from build123d import *

# Parameters (mm, degrees)
SKETCH1_R                      = 25
BOSS_EXTRUDE1_DEPTH            = 10.8
BOSS_EXTRUDE2_START            = 2
SKETCH2_R                      = 31.25
BOSS_EXTRUDE2_DEPTH            = 2
BOSS_EXTRUDE3_START            = 2.5
SKETCH3_R                      = 31.25
SKETCH3_R_2                    = 30.1
SKETCH3_R_3                    = 19.9
BOSS_EXTRUDE3_DEPTH            = 2.5
CUT_EXTRUDE1_START             = -0.4
SKETCH4_R                      = 31.25
SKETCH4_R_2                    = 27.4
CUT_EXTRUDE1_DEPTH             = 0.4
CUT_EXTRUDE2_START             = -2.5
SKETCH5_R                      = 25
SKETCH5_R_2                    = 19.9
CUT_EXTRUDE2_DEPTH             = 2.5
FILLET1_R                      = 0.2
CUT_EXTRUDE3_REACH             = 67.733
SKETCH7_R                      = 2.15
CUT_EXTRUDE3_DIRECTION_2_DEPTH = 66.732526195
CUT_EXTRUDE4_DEPTH             = 66.732526212
CUT_EXTRUDE4_DEPTH_BACK        = 16
SKETCH8_R                      = 4.15


with BuildPart() as part:
    # Sketch1 → Boss-Extrude1 (new body)
    with BuildSketch(Plane(origin=(0, 0, 0), x_dir=(1, 0, 0), z_dir=(0, 1, 0))):
        with Locations(Location((0, 0, 0), (0, 0, 90))):
            Circle(SKETCH1_R)
        with BuildLine():
            Line((-2.5, 2), (0.5, 2))
            ThreePointArc((0.5, 2), (-1, -2.5), (-2.5, 2))
        make_face(mode=Mode.SUBTRACT)
    extrude(amount=BOSS_EXTRUDE1_DEPTH)

    # Sketch2 → Boss-Extrude2 (add)
    with BuildSketch(Plane.XZ.offset(BOSS_EXTRUDE2_START)):
        with Locations(Location((-1, 0, 0), (0, 0, 270))):
            Circle(SKETCH2_R)
        with BuildLine():
            Line((0.5, -2), (-2.5, -2))
            ThreePointArc((-2.5, -2), (-1, 2.5), (0.5, -2))
        make_face(mode=Mode.SUBTRACT)
    extrude(amount=-BOSS_EXTRUDE2_DEPTH)

    # Sketch3 → Boss-Extrude3 (add)
    # profile 1 of 2: a face of its own
    with BuildSketch(Plane.XZ.offset(2).offset(BOSS_EXTRUDE3_START)):
        with Locations(Location((-1, 0, 0), (0, 0, 270))):
            Circle(SKETCH3_R)
        with Locations(Location((-1, 0, 0), (0, 0, 270))):
            Circle(SKETCH3_R_2, mode=Mode.SUBTRACT)
    # profile 2 of 2: a face of its own
    with BuildSketch(Plane.XZ.offset(2).offset(BOSS_EXTRUDE3_START)):
        with Locations(Location((-1, 0, 0), (0, 0, 270))):
            Circle(SKETCH3_R_3)
        with BuildLine():
            Line((0.5, -2), (-2.5, -2))
            ThreePointArc((-2.5, -2), (-1, 2.5), (0.5, -2))
        make_face(mode=Mode.SUBTRACT)
    extrude(amount=-BOSS_EXTRUDE3_DEPTH)

    # Sketch4 → Cut-Extrude1 (cut)
    with BuildSketch(Plane(origin=(0, 0, 0), x_dir=(1, 0, 0), z_dir=(0, 1, 0)).offset(CUT_EXTRUDE1_START)):
        with Locations(Location((-1, 0, 0), (0, 0, 270))):
            Circle(SKETCH4_R)
        with Locations(Location((0, 0, 0), (0, 0, 270))):
            Circle(SKETCH4_R_2, mode=Mode.SUBTRACT)
    extrude(amount=CUT_EXTRUDE1_DEPTH, mode=Mode.SUBTRACT)

    # Sketch5 → Cut-Extrude2 (cut)
    with BuildSketch(Plane(origin=(0, 10.8, 0), x_dir=(1, 0, 0), z_dir=(0, 1, 0)).offset(CUT_EXTRUDE2_START)):
        with Locations(Location((0, 0, 0), (0, 0, 90))):
            Circle(SKETCH5_R)
        with Locations(Location((-1, 0, 0), (0, 0, 90))):
            Circle(SKETCH5_R_2, mode=Mode.SUBTRACT)
    extrude(amount=CUT_EXTRUDE2_DEPTH, mode=Mode.SUBTRACT)

    # Sketch6 → Cut-Revolve1 (revolve, cut)
    with BuildSketch(Plane.XY, mode=Mode.PRIVATE) as cut_revolve1_sk:
        Polygon((-25, 0), (-25, 0.6), (-24.4, 0), align=None)
    revolve(cut_revolve1_sk.sketch.rotate(Axis((0, 8.3, 0), (0, -1, 0)), 90), axis=Axis((0, 8.3, 0), (0, -1, 0)), mode=Mode.SUBTRACT)

    # Fillet1
    fillet1_edges = [part.edges().sort_by_distance(p)[0] for p in [
        (0, 0, 24.4),
    ]]
    fillet(fillet1_edges, radius=FILLET1_R)

    # Sketch7 → Cut-Extrude3 (cut, up to next)
    with BuildSketch(Plane(origin=(0, 0, -25), x_dir=(-1, 0, 0), z_dir=(0, 0, -1)), mode=Mode.PRIVATE) as cut_extrude3_sk1:
        with Locations((1, 3.15)):
            Circle(SKETCH7_R)
    cut_extrude3_tool1 = extrude(cut_extrude3_sk1.sketch, amount=-CUT_EXTRUDE3_REACH, mode=Mode.PRIVATE) & part.part
    add(cut_extrude3_tool1.solids().sort_by_distance((-1, 3.15, -25))[0], mode=Mode.SUBTRACT)

    # Sketch7 → Cut-Extrude3 direction 2 (cut)
    with BuildSketch(Plane(origin=(0, 0, -25), x_dir=(-1, 0, 0), z_dir=(0, 0, -1))):
        with Locations((1, 3.15)):
            Circle(SKETCH7_R)
    extrude(amount=CUT_EXTRUDE3_DIRECTION_2_DEPTH, mode=Mode.SUBTRACT)

    # Sketch8 → Cut-Extrude4 (cut, two sides: drawn at the far end of the back side and taken through both)
    with BuildSketch(Plane(origin=(0, 0, -25), x_dir=(-1, 0, 0), z_dir=(0, 0, -1)).offset(-CUT_EXTRUDE4_DEPTH_BACK)):
        with Locations(Location((1, 3.15, 0), (0, 0, 217.912535811))):
            Circle(SKETCH8_R)
    extrude(amount=CUT_EXTRUDE4_DEPTH + CUT_EXTRUDE4_DEPTH_BACK, mode=Mode.SUBTRACT)


solid = part.part
Could you check a few things on this model? Use its own coordinates, in mm. A direction names the side the tool comes from. Coordinates: 2 decimals unless noted, no trailing zeros. Order: outer loops, then holes, each group sorted by start corner. A loop starts at its lowest first (then second) coordinate and runs counter-clockwise, first axis right, second up. Notation, with made-up numbers: (88.5, 7) -> (104.5, 7) arc R7 cw to (104.5, 16) -> close; hole circle Ø1 at (19.5, -14). An arc over 180 degrees is marked (long way). One line per item, written item: value. Start each with the question number.
1) We'd pull the mould along Z, two halves only. Please class faces 1 (the flat face through (-1, -1, -2)), 2 (the cylindrical face through (-13.1, -3.3, 15.8)), 3 (the flat face through (2, 3, -9)), 4 (the cylindrical face through (-1, -1, -17)): +Z half, -Z half, draft (parallel to the pull), parting line (faces both ways), or undercut.
2) Which directions (+Z, -Z, +X, -X, +Y, -Y) give clear straight access to the entire face, cutting with the end or side of a thin tool? Please do faces 5 (the flat face through (18.4, 8.3, -5.4)), 6 (the cylindrical face through (-3.05, 3.8, -5.19)), 7 (the flat face through (-1, 8, -2)), 8 (the conical face through (2.061, 0.469, 24.783)), 9 (the flat face through (-21, -2, -6)).
3) Imagine slicing it at D-D on x = -1. Count the separate pieces of the cut face and the enclosed holes in it, plus the area to 3 significant figures.
4) If I drill on L1, parallel to X at y = -3, z = -1; L2, parallel to X at y = -1.1, z = 0; L3, parallel to X at y = -3.25, z = 14.5, over which ranges is the centre line in solid material (lowest first)? Write a range as [from, to].
5) I'm going to push flat-ended pins straight in: pin 1 (3 mm diameter, centred on x = 1.5, y = 8, fed in from -Z); pin 2 (5.5 mm diameter, centred on x = -1, y = 3.15, fed in from -Z); pin 3 (3 mm diameter, centred on x = 8.5, y = 7.5, fed in from +Z). Where does each tip first touch, or does it pass through?
6) Imagine slicing it at C-C on y = 3.15. List the corners of the cut face in (x, z) for me.
7) Imagine slicing it at B-B on x = -26.5. List the corners of the cut face in (y, z) for me, plus the area to 3 significant figures.
Answer list:
1. face 1: undercut
1. face 2: undercut
1. face 3: -Z half
1. face 4: draft
2. face 5: +Y
2. face 6: -Z
2. face 7: +Y, -Y
2. face 8: none
2. face 9: -Y
3. separate pieces: 3
3. enclosed holes: 0
3. area: 505 mm2
4. L1: x = [-32.23, -31.08], [-20.87, -3.29], [1.29, 18.87], [29.08, 30.23]
4. L2: x = [-32.25, -3.5], [1.5, 30.25]
4. L3: x = [-28.68, -27.38], [-14.63, 12.63], [25.38, 26.68]
5. pin 1: stops at z = -25
5. pin 2: stops at z = -9
5. pin 3: stops at z = 24
6. outline: (-5.15, -24.46) -> (-5.15, -9) -> (-3.15, -9) -> (-3.15, -1.28) arc R2.5 cw (long way) to (1.15, -1.28) -> (1.15, -9) -> (3.15, -9) -> (3.15, -24.8) arc R25 ccw (long way) to start
7. outline: (-4.5, -18.06) -> (-0.4, -18.06) -> (-0.4, -6.96) -> (0, -6.96) -> (0, 6.96) -> (-0.4, 6.96) -> (-0.4, 18.06) -> (-4.5, 18.06) -> (-4.5, 15.99) -> (-2, 15.99) -> (-2, -15.99) -> (-4.5, -15.99) -> close
7. area: 73.7 mm2
